```python
from build123d import *

# Parameters (mm, degrees)
SKETCH1_W           = 141
SKETCH1_H           = 80
BOSS_EXTRUDE1_DEPTH = 6
SKETCH2_W           = 20
SKETCH2_H           = 6
BOSS_EXTRUDE2_DEPTH = 6
SKETCH3_W           = 20
SKETCH3_H           = 6
BOSS_EXTRUDE3_DEPTH = 6
SKETCH4_W           = 15
SKETCH4_H           = 6
BOSS_EXTRUDE4_DEPTH = 6
SKETCH5_W           = 20
SKETCH5_H           = 6
BOSS_EXTRUDE5_DEPTH = 6
CUT_EXTRUDE1_DEPTH  = 6


with BuildPart() as part:
    # Sketch1 → Boss-Extrude1 (new body)
    with BuildSketch(Plane(origin=(0, 0, 0), x_dir=(1, 0, 0), z_dir=(0, 1, 0))):
        with Locations((70.5, -40)):
            Rectangle(SKETCH1_W, SKETCH1_H)
    extrude(amount=BOSS_EXTRUDE1_DEPTH)

    # Sketch2 → Boss-Extrude2 (add)
    with BuildSketch(Plane.XY.offset(80)):
        with Locations((40, 3)):
            Rectangle(SKETCH2_W, SKETCH2_H)
        with Locations((101, 3)):
            Rectangle(SKETCH2_W, SKETCH2_H)
    extrude(amount=BOSS_EXTRUDE2_DEPTH)

    # Sketch3 → Boss-Extrude3 (add)
    with BuildSketch(Plane(origin=(0, 0, 0), x_dir=(-1, 0, 0), z_dir=(0, 0, -1))):
        with Locations((-101, 3)):
            Rectangle(SKETCH3_W, SKETCH3_H)
        with Locations((-40, 3)):
            Rectangle(SKETCH3_W, SKETCH3_H)
    extrude(amount=BOSS_EXTRUDE3_DEPTH)

    # Sketch4 → Boss-Extrude4 (add)
    with BuildSketch(Plane.ZY):
        with Locations((17.5, 3)):
            Rectangle(SKETCH4_W, SKETCH4_H)
        with Locations((62.5, 3)):
            Rectangle(SKETCH4_W, SKETCH4_H)
    extrude(amount=BOSS_EXTRUDE4_DEPTH)

    # Sketch5 → Boss-Extrude5 (add)
    with BuildSketch(Plane(origin=(141, 0, 0), x_dir=(0, 0, -1), z_dir=(1, 0, 0))):
        with Locations((-40, 3)):
            Rectangle(SKETCH5_W, SKETCH5_H)
    extrude(amount=BOSS_EXTRUDE5_DEPTH)

    # Sketch6 → Cut-Extrude1 (cut)
    with BuildSketch(Plane(origin=(0, 6, 0), x_dir=(1, 0, 0), z_dir=(0, 1, 0))):
        with BuildLine():
            Line((0, -25), (3, -25))
            ThreePointArc((3, -25), (7.242640687, -26.757359313), (9, -31))
            Line((9, -31), (9, -49))
            ThreePointArc((9, -49), (7.242640687, -53.242640687), (3, -55))
            Line((3, -55), (0, -55))
            Line((0, -55), (0, -25))
        make_face()
    extrude(amount=-CUT_EXTRUDE1_DEPTH, mode=Mode.SUBTRACT)


solid = part.part
```
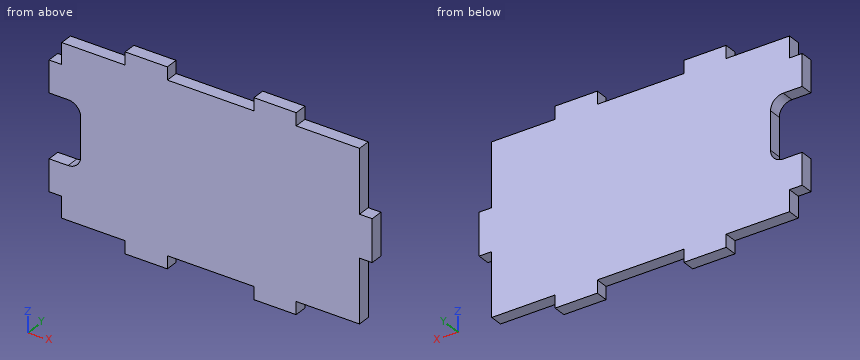
For this review, take the finished solid that the model builds, in its own axes (mm). Coordinates: 2 decimals unless noted, no trailing zeros. Write each loop counter-clockwise with the first axis right and the second up, starting at its lowest first coordinate (ties: lowest second). Pieces come first, ordered by that corner, then holes.
(1) Add section C-C on z = 77. Give the boundary of the cut face in (x, y), then the cut area to 3 significant figures.
(2) Add section B-B on x = 85.5. Give the boundary of the cut face in (y, z).
(3) Wall thickness on probe 1 along Z at (x, y) = (18.5, 3.55); probe 2 along X at (y, z) = (3.3, 20); probe 3 along X at (y, z) = (4.5, 33): over which ranges is each line inside the solid? List them lowest first.
(4) For pin 1 Ø1.5 at (x, y) = (131.5, 5) entering from -Z; pin 2 Ø3 at (y, z) = (4.5, 50) entering from -X; pin 3 Ø1.8 at (y, z) = (2, 82) entering from +X; pin 4 Ø2 at (x, z) = (73, 72.5) entering from -Y, all flat-tipped, find the tip position at first contact; note any pin that passes through.
Answer sheet:
1. outline: (0, 0) - (141, 0) - (141, 6) - (0, 6) - close
1. area: 846 mm2
2. outline: (0, 0) - (6, 0) - (6, 80) - (0, 80) - close
3. probe 1: z = 0 to 80
3. probe 2: x = -6 to 141
3. probe 3: x = 9 to 147
4. pin 1: stops at z = 0
4. pin 2: stops at x = 8.45
4. pin 3: stops at x = 111
4. pin 4: stops at y = 0
